Autodesk Inventor part; units mm, degrees
ref_plane "YZ Plane" through (0, 0, 0) normal (1, 0, 0) x (0, 1, 0)
ref_plane "XZ Plane" through (0, 0, 0) normal (0, 1, 0) x (-1, 0, 0)
ref_plane "XY Plane" through (0, 0, 0) normal (0, 0, 1) x (1, 0, 0)
sketch "Sketch1" plane through (0, 0, 0) normal (0, 1, 0) x (-1, 0, 0)
  line L0 (0, 0) -> (0, -1219.2)
  line L1 (0, 0) -> (88.9, 0)
  line L2 (88.9, 0) -> (88.9, -1219.2)
  line L3 (88.9, -1219.2) -> (0, -1219.2)
  line L4 (0, 0) -> (0, 1219.2) construction
  line L5 (0, 1219.2) -> (1219.2, 1219.2) construction
  line L6 (0, 1219.2) -> (0, 3657.6) construction
  line L7 (0, 3657.6) -> (0, 4876.8) construction
  line L8 (0, 4876.8) -> (0, 6096) construction
  line L9 (0, -1219.2) -> (2438.4, -1219.2) construction
  line L10 (0, 6096) -> (2438.4, 6096) construction
  line L11 (2438.4, 6096) -> (2438.4, -1219.2) construction
  line L12 (0, 3657.6) -> (0, 3352.8) construction
  line L13 (0, 3352.8) -> (2438.4, 3352.8) construction
  line L14 (2438.4, 3352.8) -> (1219.2, 3352.8)
  line L15 (1219.2, 3352.8) -> (1219.2, 3263.9)
  line L16 (1219.2, 3263.9) -> (2438.4, 3263.9)
  line L17 (2438.4, 3263.9) -> (2438.4, 3352.8)
  line L18 (0, 6096) -> (862.1046, 6958.1046)
  line L19 (862.1046, 6958.1046) -> (924.9664, 6895.2428)
  line L20 (924.9664, 6895.2428) -> (62.8618, 6033.1382)
  line L21 (62.8618, 6033.1382) -> (0, 6096)
  line L22 (0, 4876.8) -> (1219.2, 4876.8) construction
  line L23 (1219.2, 4876.8) -> (2081.3046, 5738.9046)
  line L24 (1219.2, 1219.2) -> (2081.3046, 357.0954)
  line L25 (2081.3046, 357.0954) -> (2018.4428, 294.2336)
  line L26 (2018.4428, 294.2336) -> (1156.3382, 1156.3382)
  line L27 (1156.3382, 1156.3382) -> (1219.2, 1219.2)
  line L28 (2018.4428, 294.2336) -> (88.9, -1219.2)
  line L29 (2081.3046, 357.0954) -> (2144.1664, 419.9572)
  line L30 (2144.1664, 419.9572) -> (1282.0618, 1282.0618)
  line L31 (1282.0618, 1282.0618) -> (1219.2, 1219.2)
  line L32 (2438.4, 3352.8) -> (2438.4, 3441.7)
  line L33 (2438.4, 3441.7) -> (1219.2, 3441.7)
  line L34 (1219.2, 3441.7) -> (1219.2, 3352.8)
  line L35 (1156.3382, 4939.6618) -> (1282.0618, 4813.9382)
  line L36 (2018.4428, 5801.7664) -> (2144.1664, 5676.0428)
  line L37 (1282.0618, 4813.9382) -> (2144.1664, 5676.0428)
  line L38 (2018.4428, 5801.7664) -> (1156.3382, 4939.6618)
  line L39 (2018.4428, 5801.7664) -> (924.9664, 6895.2428)
  line L40 (62.8618, 6033.1382) -> (1156.3382, 4939.6618)
  line L41 (1233.6206, 4168.8855) -> (1267.6412, 4086.7527)
  line L42 (1263.7078, 2313.9849) -> (1230.0006, 2231.7229)
  arc A0 (862.1046, 6958.1046) -> (0, 6096) centre (431.0523, 6527.0523) ccw
  line L43 (1246.8542, 2272.8539) -> (2375.0183, 1810.583)
  line L44 (2391.8719, 1851.7139) -> (2358.1646, 1769.452)
  line L45 (2391.8719, 1851.7139) -> (1263.7078, 2313.9849)
  line L46 (1230.0006, 2231.7229) -> (2358.1646, 1769.452)
  line L47 (1230.0006, 2231.7229) -> (1219.2, 3263.9)
  line L48 (2144.1664, 419.9572) -> (2391.8719, 1851.7139)
  line L49 (2391.8719, 1851.7139) -> (2438.4, 3263.9)
  line L50 (1219.2, 3441.7) -> (1233.6206, 4168.8855)
  line L51 (1250.6309, 4127.8191) -> (2377.0248, 4594.3867)
  line L52 (2360.0145, 4635.4532) -> (2394.0351, 4553.3203)
  line L53 (2394.0351, 4553.3203) -> (1267.6412, 4086.7527)
  line L54 (2360.0145, 4635.4532) -> (1233.6206, 4168.8855)
  line L55 (2394.0351, 4553.3203) -> (2144.1664, 5676.0428)
  line L56 (2438.4, 3441.7) -> (2394.0351, 4553.3203)
  line L57 (2144.1664, 5676.0428) -> (2057.3895, 5656.7301)
  line L58 (2394.0351, 4553.3203) -> (2305.2058, 4549.7751)
  line L59 (2394.0351, 4553.3203) -> (2307.2582, 4534.0076)
  line L60 (2307.2582, 4534.0076) -> (2057.3895, 5656.7301)
  line L61 (2438.4, 3441.7) -> (2349.5707, 3438.1548)
  line L62 (2349.5707, 3438.1548) -> (2305.2058, 4549.7751)
  line L63 (1219.2, 3441.7) -> (1308.0825, 3439.9374)
  line L64 (1233.6206, 4168.8855) -> (1322.5031, 4167.1229)
  line L65 (1322.5031, 4167.1229) -> (1308.0825, 3439.9374)
  line L66 (2018.4428, 5801.7664) -> (1955.581, 5738.9046)
  line L67 (1955.581, 5738.9046) -> (862.1046, 6832.381)
  line L68 (924.9664, 6895.2428) -> (862.1046, 6832.381)
  line L69 (62.8618, 6033.1382) -> (125.7236, 6096)
  line L70 (62.8618, 6033.1382) -> (125.7236, 6096)
  line L71 (125.7236, 6096) -> (1219.2, 5002.5236)
  line L72 (1156.3382, 1156.3382) -> (0, 0)
  line L73 (0, 0) -> (62.8618, -62.8618)
  line L74 (1156.3382, 1156.3382) -> (1219.2, 1093.4764)
  line L75 (1219.2, 1093.4764) -> (62.8618, -62.8618)
  line L76 (2018.4428, 294.2336) -> (1963.5776, 364.1837)
  line L77 (88.9, -1219.2) -> (34.0348, -1149.2499)
  line L78 (34.0348, -1149.2499) -> (1963.5776, 364.1837)
  line L79 (2144.1664, 419.9572) -> (2056.5677, 435.1125)
  line L80 (2391.8719, 1851.7139) -> (2304.2732, 1866.8692)
  line L81 (2391.8719, 1851.7139) -> (2303.0201, 1854.6414)
  line L82 (2304.2732, 1866.8692) -> (2056.5677, 435.1125)
  line L83 (1230.0006, 2231.7229) -> (1318.8957, 2232.6531)
  line L84 (1219.2, 3263.9) -> (1308.0951, 3264.8302)
  line L85 (1308.0951, 3264.8302) -> (1318.8957, 2232.6531)
  line L86 (2438.4, 3263.9) -> (2349.5482, 3266.8275)
  line L87 (2349.5482, 3266.8275) -> (2303.0201, 1854.6414)
  line L88 (88.9, 0) -> (125.7236, 0)
  line L89 (1233.6206, 4168.8855) -> (1219.2, 4876.8)
  line L90 (1233.6206, 4168.8855) -> (1322.5022, 4170.6961)
  line L91 (1219.2, 4876.8) -> (1308.0816, 4878.6106)
  line L92 (1308.0816, 4878.6106) -> (1322.5022, 4170.6961)
  line L93 (1282.0618, 4813.9382) -> (1309.9674, 4786.0326)
  line L94 (1267.6412, 4086.7527) -> (1318.4756, 3964.0275)
  line L95 (2360.0145, 4635.4532) -> (2374.4273, 4641.4231)
  line L96 (1230.0006, 2231.7229) -> (1219.2, 1219.2)
  line L97 (1230.0006, 2231.7229) -> (1318.8955, 2230.7747)
  line L98 (1219.2, 1219.2) -> (1308.0949, 1218.2518)
  line L99 (1308.0949, 1218.2518) -> (1318.8955, 2230.7747)
  line L100 (1282.0618, 1282.0618) -> (1309.0636, 1309.0636)
  line L101 (1263.7078, 2313.9849) -> (1316.7428, 2438.4)
  line L102 (2358.1646, 1769.452) -> (2376.5379, 1763.082)
  point P0 (1770.957, 2057.4547)
  point P1 (1955.1236, 357.5528)
  point P2 (88.9, -1106.2164)
  point P3 (2292.1025, 1796.5213)
  point P4 (2067.2525, 496.8711)
  point P5 (1318.5187, 2195.4522)
  point P6 (1308.1049, 3263.9)
  point P7 (2349.4518, 3263.9)
  point P8 (2304.1085, 1887.6754)
  dimension "d0" = 1219.2
  dimension "d2" = 1219.2
  dimension "d3" = 1219.2
  dimension "d16" = 2438.4
  dimension "d17" = 1219.2
  dimension "d18" = 1219.2
  dimension "d20" = 2438.4
  dimension "d21" = 304.8
  dimension "d22" = 1219.2
  dimension "d23" = 88.9
  dimension "d24" = 1219.2
  dimension "d25" = 45
  dimension "d26" = 88.9
  dimension "d27" = 1219.2
  dimension "d28" = 1219.2
  dimension "d29" = 1219.2
  dimension "d31" = 1219.2
  dimension "d32" = 88.9
  dimension "d33" = 88.9
  dimension "d34" = 88.9
  dimension "d35" = 177.8
  dimension "d36" = 177.8
  dimension "d38" = 88.9
  dimension "d39" = 88.9
  dimension "d43" = 1219.2
  dimension "d44" = 88.9
  dimension "d45" = 1219.2
  dimension "d46" = 88.9
  dimension "d47" = 88.9
  dimension "d48" = 88.9
  dimension "d49" = 88.9
  dimension "d50" = 88.9
  dimension "d51" = 88.9
  dimension "d54" = 88.9
  dimension "d55" = 88.9
  dimension "d57" = 88.9
  dimension "d58" = 88.9
  dimension "d59" = 88.9
  dimension "d60" = 88.9
  dimension "d61" = 88.9
  dimension "d64" = 88.9
  dimension "d65" = 88.9
  dimension "d66" = 88.9
  dimension "d69" = 88.9
  dimension "d70" = 88.9
  dimension "d71" = 88.9
  dimension "d72" = 88.9
extrude "Extrusion1" add sketch "Sketch1" along normal blind 38.1 contours L47 L16 L85 L101 L42
properties part number "S_2x4x40.639"
CAD build for the part. Positions are in the model's coordinates, mm. Coordinates: 2 decimals unless noted, no trailing zeros. Write each loop counter-clockwise with the first axis right and the second up, starting at its lowest first coordinate (ties: lowest second). Pieces come first, ordered by that corner, then holes. Notation, with made-up numbers: M 50.5,55 L 92.5,55 A26 ccw 92.5,85 Z; hole C 82.25,78 d1. An arc over 180 degrees is marked long. Return JSON: item names as keys, results as strings.
Item 1: Slice it at A-A, the plane y = 28. Write the cut outline in (x, z).
Findings below:
{"outline": "M -1316.74,2438.4 L -1263.71,2313.98 L -1230,2231.72 L -1219.2,3263.9 L -1308.1,3263.9 Z"}
Item 2: Slice it at C-C, the plane z = 3197. Write the cut outline in (x, y).
Findings below:
{"outline": "M -1308.8,0 L -1219.9,0 L -1219.9,38.1 L -1308.8,38.1 Z"}
Item 3: Slice it at B-B, the plane x = -1288. Write the cut outline in (y, z).
Findings below:
{"outline": "M 0,2370.97 L 38.1,2370.97 L 38.1,3263.9 L 0,3263.9 Z"}
Item 4: Probe line 1 (Z direction, x = -1248, y = 11.5); line 2 (X direction, y = 31.5, z = 2780.5); line 3 (Z direction, x = -1294, y = 28.5). List the from-to ranges inside material, lowest first. Write a range as from..to.
Findings below:
{"line 1": "z = 2275.65..3263.9", "line 2": "x = -1313.16..-1224.26", "line 3": "z = 2385.05..3263.9"}
Item 5: Drop flat-ended pins along their axis: pin 1 Ø2 at (y, z) = (14.5, 2536) entering from -X; pin 2 Ø3 at (x, y) = (-1271, 7.5) entering from -Z; pin 3 Ø8 at (y, z) = (6.5, 2653) entering from +X. Give the stop position or say it passes through.
Findings below:
{"pin 1": "stops at x = -1315.73", "pin 2": "stops at z = 2327.57", "pin 3": "stops at x = -1225.55"}
